Input: part model. Units: mm. Frame: model coordinates. A direction names the side the tool comes from. Give positions to 0.01 mm unless a question says otherwise; leave off trailing zeros. Loops run counter-clockwise (first coordinate to the right, second up) from the corner with the lowest first, then second, coordinate; pieces in that order, holes last. Notation, with made-up numbers: M 72,-21.5 L 118,-21.5 A15 ccw 118,6.5 Z; hole C -17.75,31 d11. An arc over 180 degrees is marked long. One line per item, written item: value. Start each with the question number.
(1) Section A-A on z = 12.9. Output: boundary loops of the cut face in (x, y), plus the area to 3 significant figures.
(2) Access query for faces 1 (the flat face through (2, 19, 65)), 2 (the flat face through (10, 3, 32)). Directions: +Z, -Z, +X, -X, +Y, -Y. A direction counts if a zero-diameter tool reaches every point of the face in a straight line with its end or side. Return the directions, or none.
(3) Section D-D on x = 15.5. Output: boundary loops of the cut face in (y, z), plus the area to 3 significant figures.
(4) Section B-B on y = 26. Output: boundary loops of the cut face in (x, z), plus the area to 3 significant figures.
(5) Pin query (flat end, axial travel): P1, Ø1.5, axis at y = 35.5, z = 38.5, coming from the +X side; P2, Ø3, axis at x = 7, z = 36.5, coming from the +Y side. Return the tip coordinate at first contact, or that it passes through.
(6) Section C-C on z = 28.5. Output: boundary loops of the cut face in (x, y).
(7) Pull-direction query (Z, two-part tool) for faces 3 (the flat face through (2, 19, 0)), 4 (the flat face through (18, 1, 32)), 5 (the cylindrical face through (1.5, 23.6, 11.1)); classes: released by +Z, released by -Z, zero draft, split by the parting line, or undercut.
(8) Ray query, line 1 along Z through (x, y) = (2.1, 26); line 2 along X through (y, z) = (12.5, 27). Return the intervals inside material, ascending. Write a range as from..to.
```python
from build123d import *

# Parameters (mm, degrees)
SKETCH_1_W          = 15
SKETCH_1_H          = 3
EXTRUDE_1_DEPTH     = 65
SKETCH_2_R          = 3
CUT_EXTRUDE_1_DEPTH = 64.5


with BuildPart() as part:
    # 草图1 → 凸台-拉伸1 (new body)
    with BuildSketch(Plane.XY):
        Polygon((3, 45), (0, 45), (0, 0), (3, 0), (3, 3), align=None)
        with Locations((10.5, 1.5)):
            Rectangle(SKETCH_1_W, SKETCH_1_H)
    extrude(amount=EXTRUDE_1_DEPTH)

    # 草图2 → 切除-拉伸1 (cut)
    with BuildSketch(Plane(origin=(3, 0, 0), x_dir=(0, 0, -1), z_dir=(1, 0, 0))):
        with Locations(Location((-12.9, 26, 0), (0, 0, 90))):
            Circle(SKETCH_2_R)
    extrude(amount=-CUT_EXTRUDE_1_DEPTH, mode=Mode.SUBTRACT)


solid = part.part
```
Output values:
1. outline: M 0,0 L 18,0 L 18,3 L 3,3 L 3,23 L 0,23 Z; M 0,29 L 3,29 L 3,45 L 0,45 Z
1. area: 162 mm²
2. face 1: +Z, +X, -X, +Y, -Y
2. face 2: +Z, -Z, +X, +Y
3. outline: M 0,0 L 3,0 L 3,65 L 0,65 Z
3. area: 195 mm²
4. outline: M 0,0 L 3,0 L 3,9.9 L 0,9.9 Z; M 0,15.9 L 3,15.9 L 3,65 L 0,65 Z
4. area: 177 mm²
5. P1: stops at x = 3
5. P2: stops at y = 3
6. outline: M 0,0 L 18,0 L 18,3 L 3,3 L 3,45 L 0,45 Z
7. face 3: released by -Z
7. face 4: zero draft
7. face 5: undercut
8. line 1: z = 0..9.9, 15.9..65
8. line 2: x = 0..3
